CAD build for the part. Positions are in the model's coordinates, mm. A direction names the side the tool comes from. Give positions to 0.01 mm unless a question says otherwise; leave off trailing zeros. Order: outer loops, then holes, each group sorted by start corner. A loop starts at its lowest first (then second) coordinate and runs counter-clockwise, first axis right, second up.
Item 1: Flat gauge pins, fed straight in: P1, Ø10, axis at y = 15.5, z = 18, coming from the +X side; P2, Ø6, axis at y = -13.5, z = 20.5, coming from the -X side; P3, Ø14.5, axis at x = 27.5, z = 12.5, coming from the -Y side. Where does each tip first touch, or does it go through?
Item 2: Which spindle directions (+Z, -Z, +X, -X, +Y, -Y) get a long thin tool onto all of the face, cutting with end or side? Do faces 5 (the flat face through (-23, -5, 2)), 6 (the flat face through (-10, 0, 20)), 7 (the flat face through (14, -5, 17)). Say none if no direction does.
Item 3: Band-saw the part on D-D on y = -20. Give the cut face in (x, z), plus the area to 3 significant figures.
Item 4: Wall check: L1, parallel to X at y = 28.75, z = 15; L2, parallel to Y at x = 0, z = 6.75; L3, parallel to X at y = -30, z = 23.25. Give the ranges that are in metal, low to high.
Item 5: Band-saw the part on C-C on z = 15. Give the cut face in (x, y).
Item 6: Two-plate mould, pull along Y, no slides. Class faces 1 (the cylindrical face through (12, -25, 22)), 2 (the flat face through (-19, 9, 5)), 3 (the cylindrical face through (0, -18, 5)), 4 (the flat face through (0, 35, 8)): released by +Y, released by -Y, zero draft, split by the parting line, or undercut.
Item 7: Band-saw the part on B-B on y = 5. Give the cut face in (x, z).
Item 8: Band-saw the part on A-A on x = -20. Give the cut face in (y, z), plus the area to 3 significant figures.
```python
from build123d import *

# Parameters (mm, degrees)
SKETCH_1_W          = 28
SKETCH_1_H          = 70
EXTRUDE_1_DEPTH     = 30
SKETCH_2_W          = 20
SKETCH_2_H          = 70
CUT_EXTRUDE_1_DEPTH = 20
SKETCH_4_W          = 18
SKETCH_4_H          = 30
EXTRUDE_2_DEPTH     = 10
SKETCH_5_R          = 3
CUT_EXTRUDE_2_DEPTH = 19
EXTRUDE_3_DEPTH     = 5
SKETCH_8_R          = 2
CUT_EXTRUDE_3_DEPTH = 98
SKETCH_9_R          = 2
CUT_EXTRUDE_4_DEPTH = 98


with BuildPart() as part:
    # 草图1 → 凸台-拉伸1 (new body)
    with BuildSketch(Plane.XY):
        Rectangle(SKETCH_1_W, SKETCH_1_H)
    extrude(amount=EXTRUDE_1_DEPTH)

    # 草图2 → 切除-拉伸1 (cut)
    with BuildSketch(Plane.XY.offset(30)):
        Rectangle(SKETCH_2_W, SKETCH_2_H)
    extrude(amount=-CUT_EXTRUDE_1_DEPTH, mode=Mode.SUBTRACT)

    # 草图4 → 凸台-拉伸2 (add)
    with BuildSketch(Plane(origin=(0, 35, 0), x_dir=(1, 0, 0), z_dir=(0, 1, 0))):
        with Locations((23, -15)):
            Rectangle(SKETCH_4_W, SKETCH_4_H)
    extrude(amount=-EXTRUDE_2_DEPTH)

    # 草图5 → 切除-拉伸2 (cut)
    with BuildSketch(Plane(origin=(0, 35, 0), x_dir=(1, 0, 0), z_dir=(0, 1, 0))):
        with Locations(Location((20, -15, 0), (0, 0, 270))):
            Circle(SKETCH_5_R)
    extrude(amount=-CUT_EXTRUDE_2_DEPTH, mode=Mode.SUBTRACT)

    # 草图7 → 凸台-拉伸3 (add)
    with BuildSketch(Plane(origin=(0, 0, 0), x_dir=(-1, 0, 0), z_dir=(0, 0, -1))):
        Polygon((-32, 25), (-14, -35), (-14, 25), align=None)
    extrude(amount=-EXTRUDE_3_DEPTH)

    # 镜向1: part across plane


with BuildPart() as part_1:
    add(part.part)
    add(part.part.mirror(Plane(origin=(0, 0, 0), x_dir=(0, 0, 1), z_dir=(1, 0, 0))))

    # 草图8 → 切除-拉伸3 (cut)
    with BuildSketch(Plane(origin=(14, 0, 0), x_dir=(0, 0, -1), z_dir=(1, 0, 0))):
        with Locations(Location((-20, -25, 0), (0, 0, 90))):
            Circle(SKETCH_8_R)
        with Locations(Location((-20, 5, 0), (0, 0, 90))):
            Circle(SKETCH_8_R)
    extrude(amount=-CUT_EXTRUDE_3_DEPTH, mode=Mode.SUBTRACT)

    # 草图9 → 切除-拉伸4 (cut)
    with BuildSketch(Plane.XY.offset(10)):
        with Locations((0, -20)):
            Circle(SKETCH_9_R)
        with Locations((0, 20)):
            Circle(SKETCH_9_R)
    extrude(amount=-CUT_EXTRUDE_4_DEPTH, mode=Mode.SUBTRACT)


solid = part_1.part
```
The answers:
1. P1: stops at x = 14
1. P2: stops at x = -14
1. P3: stops at y = 25
2. face 5: +Z, -Z, -X, -Y
2. face 6: +Z, +Y, -Y
2. face 7: +Z, +X, -Y
3. outline: (-18.5, 0) - (-2, 0) - (-2, 10) - (-10, 10) - (-10, 30) - (-14, 30) - (-14, 5) - (-18.5, 5) - close; (2, 0) - (18.5, 0) - (18.5, 5) - (14, 5) - (14, 30) - (10, 30) - (10, 10) - (2, 10) - close
3. area: 445 mm2
4. L1: x = -32 to -23, -17 to -10, 10 to 17, 23 to 32
4. L2: y = -35 to -22, -18 to 18, 22 to 35
4. L3: x = -14 to -10, 10 to 14
5. outline: (-32, 25) - (-23, 25) - (-23, 35) - (-32, 35) - close; (-17, 25) - (-14, 25) - (-14, -35) - (-10, -35) - (-10, 35) - (-17, 35) - close; (10, -35) - (14, -35) - (14, 25) - (17, 25) - (17, 35) - (10, 35) - close; (23, 25) - (32, 25) - (32, 35) - (23, 35) - close
6. face 1: undercut
6. face 2: zero draft
6. face 3: undercut
6. face 4: released by +Y
7. outline: (-26, 0) - (26, 0) - (26, 5) - (14, 5) - (14, 18) - (10, 18) - (10, 10) - (-10, 10) - (-10, 18) - (-14, 18) - (-14, 5) - (-26, 5) - close; (-14, 22) - (-10, 22) - (-10, 30) - (-14, 30) - close; (10, 22) - (14, 22) - (14, 30) - (10, 30) - close
8. outline: (-15, 0) - (35, 0) - (35, 12) - (25, 12) - (25, 5) - (-15, 5) - close; (25, 18) - (35, 18) - (35, 30) - (25, 30) - close
8. area: 440 mm2
